```python
from build123d import *

# Parameters (mm, degrees)
F0_W     = 35
F0_H     = 30
F1_DEPTH = 20
F2_W     = 10
F2_H     = 4
F3_DEPTH = 40
F4_R     = 1
F5_DEPTH = 25
F6_W     = 1.9774927944
F6_H     = 23.6601198859
F7_DEPTH = 20


with BuildPart() as f1:
    # F0 (on Top) → F1 (new body)
    with BuildSketch(Plane.XY):
        with Locations((-5.7433683425, -12.3615624963)):
            Rectangle(F0_W, F0_H)
    extrude(amount=F1_DEPTH)

    # F2 (on face) → F3 (cut)
    with BuildSketch(Plane.XZ.offset(27.3615624963)):
        with Locations((-18.2433683425, 10)):
            Rectangle(F2_W, F2_H)
    extrude(amount=-F3_DEPTH, mode=Mode.SUBTRACT)

    # F4 (on face) → F5 (cut)
    with BuildSketch(Plane.XY.offset(20)):
        with Locations((-18.2433683425, 3.8932797033)):
            Circle(F4_R)
        with Locations((-18.2433683425, -16.9682204723)):
            Circle(F4_R)
    extrude(amount=-F5_DEPTH, mode=Mode.SUBTRACT)

    # F6 (on face) → F7 (join)
    with BuildSketch(Plane.XY.offset(20)):
        with Locations((-22.2546219453, -15.5315025534)):
            Rectangle(F6_W, F6_H)
        Polygon((-23.2433683425, -3.7014426105), (-21.2658755481, -3.7014426105), (-21.2658755481, -27.3615624963), (11.7566316575, -27.3615624963), (11.7566316575, 2.6384375037), (-23.2433683425, 2.6384375037), align=None)
    extrude(amount=F7_DEPTH)


solid = f1.part
```
For this review, take the finished solid that the model builds, in its own axes (mm). A direction names the side the tool comes from. Coordinates: 2 decimals unless noted, no trailing zeros. Write each loop counter-clockwise with the first axis right and the second up, starting at its lowest first coordinate (ties: lowest second). Pieces come first, ordered by that corner, then holes.
(1) Tool access review of faces 1 (the face through (-6, -12, 40)), 2 (the face through (-18, -13, 12)), 3 (the face through (-18, -17, 20)): name each direction out of +Z, -Z, +X, -X, +Y, -Y from which nothing blocks a thin tool from reaching the whole face with its end or side.
(2) Add section B-B on y = -14. Give the boundary of the cut face in (x, z).
(3) Wall thickness on probe 1 along Z at (x, y) = (-18.5, -3.5); probe 2 along X at (y, z) = (-10, 9.5); probe 3 along X at (y, z) = (-17.5, 17.5): over which ranges is each line inside the solid? List them lowest first.
(4) Add section C-C on z = 10. Give the boundary of the cut face in (x, y).
(5) Add section A-A on x = -20. Give the boundary of the cut face in (y, z).
(6) The part is to be moulded in two halves that separate along X. For faces 4 (the face through (-5, 2.638, 20)), 5 (the face through (-13.243, -13, 10)), 6 (the face through (-19.242, -16.924, 4.056)), say which applies: +X half, -X half, draft (parallel to the pull), parting line (faces both ways), or undercut.
(7) For pin 1 Ø0.6 at (x, y) = (-18.5, -16.5) entering from -Z; pin 2 Ø1.2 at (y, z) = (-7.5, 10.5) entering from -X, all flat-tipped, find the tip position at first contact; note any pin that passes through.
Answer sheet:
1. face 1: +Z, +X, -X, +Y, -Y
1. face 2: -X, +Y, -Y
1. face 3: -Z
2. outline: (-23.24, 0) - (11.76, 0) - (11.76, 40) - (-23.24, 40) - (-23.24, 12) - (-13.24, 12) - (-13.24, 8) - (-23.24, 8) - close
3. probe 1: z = 0 to 8, 12 to 40
3. probe 2: x = -13.24 to 11.76
3. probe 3: x = -23.24 to -19.09, -17.4 to 11.76
4. outline: (-13.24, -27.36) - (11.76, -27.36) - (11.76, 2.64) - (-13.24, 2.64) - close
5. outline: (-27.36, 0) - (2.64, 0) - (2.64, 8) - (-27.36, 8) - close; (-27.36, 12) - (2.64, 12) - (2.64, 40) - (-27.36, 40) - close
6. face 4: draft
6. face 5: -X half
6. face 6: undercut
7. pin 1: stops at z = 20
7. pin 2: stops at x = -13.24
